The listing builds one solid part. Answer for the finished solid, in the listing's coordinates (mm). Round coordinates to 2 decimals unless told otherwise and drop trailing zeros. Write each loop counter-clockwise with the first axis right and the second up, starting at its lowest first coordinate (ties: lowest second). Pieces come first, ordered by that corner, then holes. Notation, with made-up numbers: M -11.75,76 L 19.25,76 A12 cw 19.25,87 Z; hole C 41,0 d4. An arc over 180 degrees is marked long. Write each question's results on one line, items separated by ' | '.
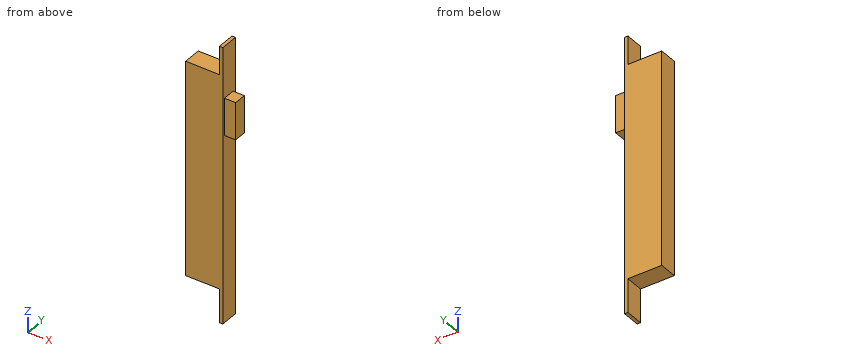
from build123d import *

# Parameters (mm, degrees)
F0_W     = 16
F0_H     = 190
F1_DEPTH = 30
F3_W     = 16
F3_H     = 245
F4_DEPTH = 3
F5_W     = 11
F5_H     = 33
F6_DEPTH = 10


with BuildPart() as f1:
    # F0 (on Right) → F1 (new body)
    with BuildSketch(Plane.YZ):
        with Locations((8, -95)):
            Rectangle(F0_W, F0_H)
    extrude(amount=F1_DEPTH)

    # F3 (on face) → F4 (join)
    with BuildSketch(Plane.YZ.offset(30)):
        with Locations((8, -97.338722)):
            Rectangle(F3_W, F3_H)
    extrude(amount=F4_DEPTH)

    # F5 (on face) → F6 (join)
    with BuildSketch(Plane.YZ.offset(33)):
        with Locations((7.497938, -37.338722)):
            Rectangle(F5_W, F5_H)
    extrude(amount=F6_DEPTH)


solid = f1.part
1) Section A-A (y = 4) is taken. Determine the outline of the cut face in (x, z).
Return value:
outline: M 0,-190 L 30,-190 L 30,-219.84 L 33,-219.84 L 33,-53.84 L 43,-53.84 L 43,-20.84 L 33,-20.84 L 33,25.16 L 30,25.16 L 30,0 L 0,0 Z
2) Section D-D (z = -113.5) is taken. Determine the outline of the cut face in (x, y), then the cut area to 3 significant figures.
Return value:
outline: M 0,0 L 33,0 L 33,16 L 0,16 Z | area: 528 mm²
3) Section B-B (z = -25.5) is taken. Determine the outline of the cut face in (x, y), then the cut area to 3 significant figures.
Return value:
outline: M 0,0 L 33,0 L 33,2 L 43,2 L 43,13 L 33,13 L 33,16 L 0,16 Z | area: 638 mm²
4) Section C-C (x = 40.5) is taken. Determine the outline of the cut face in (y, z).
Return value:
outline: M 2,-53.84 L 13,-53.84 L 13,-20.84 L 2,-20.84 Z
5) Find the intervals of material crossed by line 1 (Z direction, x = 36.5, y = 11.25); line 2 (X direction, y = 5, z = -55); line 3 (Z direction, x = 12, y = 2.75), in increasing order.
Return value:
line 1: -53.84 to -20.84 | line 2: 0 to 33 | line 3: -190 to 0
6) Each of these flat-tipped pins is pushed along its axis until it touches: pin 1 (2 mm diameter, centred on x = 35.5, y = 3.5, fed in from +Z); pin 2 (5 mm diameter, centred on x = 38, y = 5.5, fed in from -Z); pin 3 (12 mm diameter, centred on x = 23.5, z = -181, fed in from -Y); pin 4 (4 mm diameter, centred on x = 14.5, y = 8.5, fed in from +Z). Where does it stop, or does it pass through?
Return value:
pin 1: z = -20.84 | pin 2: z = -53.84 | pin 3: y = 0 | pin 4: z = 0
